```python
from build123d import *

# Parameters (mm, degrees)
CROQUIS2_W              = 65
CROQUIS2_H              = 65
CROQUIS2_R              = 15
CROQUIS2_R_2            = 4
SALIENTE_EXTRUIR1_DEPTH = 32
CROQUIS3_R              = 15
CROQUIS3_R_2            = 13.5
SALIENTE_EXTRUIR2_DEPTH = 7
REDONDEO1_R             = 1


with BuildPart() as part:
    # Croquis2 → Saliente-Extruir1 (new body)
    with BuildSketch(Plane(origin=(0, 0, 0), x_dir=(1, 0, 0), z_dir=(0, 1, 0))):
        Rectangle(CROQUIS2_W, CROQUIS2_H)
        with Locations(Location((0, 0, 0), (0, 0, 270))):
            Circle(CROQUIS2_R, mode=Mode.SUBTRACT)
        with Locations(Location((-27, 0, 0), (0, 0, 270))):
            Circle(CROQUIS2_R_2, mode=Mode.SUBTRACT)
        with Locations(Location((27, 0, 0), (0, 0, 270))):
            Circle(CROQUIS2_R_2, mode=Mode.SUBTRACT)
        with Locations(Location((0, 27, 0), (0, 0, 270))):
            Circle(CROQUIS2_R_2, mode=Mode.SUBTRACT)
        with Locations(Location((0, -27, 0), (0, 0, 270))):
            Circle(CROQUIS2_R_2, mode=Mode.SUBTRACT)
    extrude(amount=SALIENTE_EXTRUIR1_DEPTH)

    # Croquis3 → Saliente-Extruir2 (add)
    with BuildSketch(Plane(origin=(0, 0, 0), x_dir=(1, 0, 0), z_dir=(0, 1, 0))):
        with Locations(Location((0, 0, 0), (0, 0, 270))):
            Circle(CROQUIS3_R)
        with Locations(Location((0, 0, 0), (0, 0, 270))):
            Circle(CROQUIS3_R_2, mode=Mode.SUBTRACT)
    extrude(amount=SALIENTE_EXTRUIR2_DEPTH)

    # Redondeo1
    redondeo1_edges = [part.edges().sort_by_distance(p)[0] for p in [
        (-32.5, 16, -32.5),
        (32.5, 16, -32.5),
        (32.5, 16, 32.5),
        (-32.5, 16, 32.5),
    ]]
    fillet(redondeo1_edges, radius=REDONDEO1_R)


solid = part.part
```
Build history of the part. All positions in model axes, mm. A direction names the side the tool comes from. Round coordinates to 2 decimals unless told otherwise and drop trailing zeros. Loops run counter-clockwise (first coordinate to the right, second up) from the corner with the lowest first, then second, coordinate; pieces in that order, holes last.
Item 1: Saw through at D-D (z = 0). List the corners of the cut face in (x, y), then the cut area to 3 significant figures.
Item 2: Saw through at C-C (y = 25). List the corners of the cut face in (x, z).
Item 3: Saw through at A-A (z = -27). List the corners of the cut face in (x, y), then the cut area to 3 significant figures.
Item 4: Drill centre lines: line 1 along X through (y, z) = (25, 0); line 2 along X through (y, z) = (12, 27); line 3 along Z through (x, y) = (9.5, 16). Where is each one in solid material? Low to high.
Item 5: Two-plate mould, pull along X, no slides. Class faces 1 (the face through (7.85, 7, -11.18)), 2 (the face through (-32.5, 16, 0)), 3 (the face through (-15, 32, -8)): released by +X, released by -X, zero draft, split by the parting line, or undercut.
Item 6: Which spindle directions (+Z, -Z, +X, -X, +Y, -Y) get a long thin tool onto all of the face, cutting with end or side? Do faces 4 (the face through (30.966, 15.776, -0.521)), 5 (the face through (0.66, 19.325, -14.985)). Say none if no direction does.
Item 7: Pin check, flat tip, straight feed: P1, Ø9, axis at x = 0, z = 27, coming from the -Y side. Stop position of the tip, or through.
Item 8: Saw through at B-B (x = 27). List the corners of the cut face in (y, z).
Worked answers:
1. outline: (-32.5, 0) - (-31, 0) - (-31, 32) - (-32.5, 32) - close; (-23, 0) - (-13.5, 0) - (-13.5, 7) - (-15, 7) - (-15, 32) - (-23, 32) - close; (13.5, 0) - (23, 0) - (23, 32) - (15, 32) - (15, 7) - (13.5, 7) - close; (31, 0) - (32.5, 0) - (32.5, 32) - (31, 32) - close
1. area: 629 mm2
2. outline: (-32.5, -31.5) arc R1 ccw to (-31.5, -32.5) - (31.5, -32.5) arc R1 ccw to (32.5, -31.5) - (32.5, 31.5) arc R1 ccw to (31.5, 32.5) - (-31.5, 32.5) arc R1 ccw to (-32.5, 31.5) - close; hole circle Ø8 at (-27, 0); hole circle Ø30 at (0, 0); hole circle Ø8 at (0, -27); hole circle Ø8 at (0, 27); hole circle Ø8 at (27, 0)
3. outline: (-32.5, 0) - (-4, 0) - (-4, 32) - (-32.5, 32) - close; (4, 0) - (32.5, 0) - (32.5, 32) - (4, 32) - close
3. area: 1,820 mm2
4. line 1: x = -32.5 to -31, -23 to -15, 15 to 23, 31 to 32.5
4. line 2: x = -32.5 to -4, 4 to 32.5
4. line 3: z = -32.5 to -11.61, 11.61 to 32.5
5. face 1: undercut
5. face 2: released by -X
5. face 3: zero draft
6. face 4: +Y, -Y
6. face 5: +Y
7. P1: stops at y = 0
8. outline: (0, -32.5) - (32, -32.5) - (32, -4) - (0, -4) - close; (0, 4) - (32, 4) - (32, 32.5) - (0, 32.5) - close
